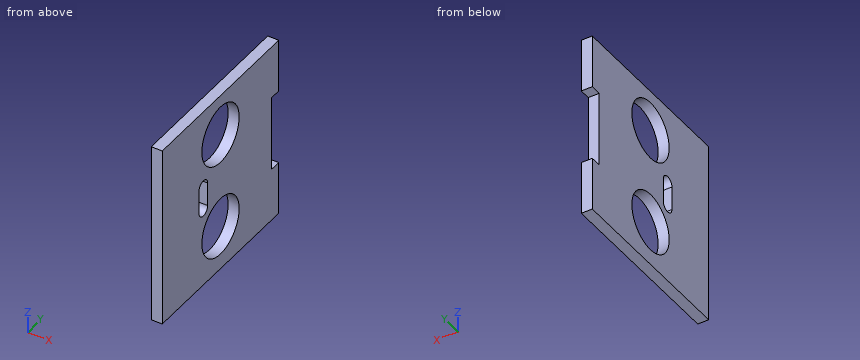
```python
from build123d import *

# Parameters (mm, degrees)
BOSS_EXTRUDE1_DEPTH = 3
SKETCH2_R           = 8
CUT_EXTRUDE1_DEPTH  = 36.482389998


with BuildPart() as part:
    # Sketch1 → Boss-Extrude1 (new body)
    with BuildSketch(Plane(origin=(0, 0, 0), x_dir=(0, 0, -1), z_dir=(1, 0, 0))):
        Polygon((-25, 25), (-10.35, 25), (-10.35, 22), (10.35, 22), (10.35, 25), (25, 25), (25, -25), (-25, -25), align=None)
    extrude(amount=BOSS_EXTRUDE1_DEPTH)

    # Sketch2 → Cut-Extrude1 (cut, through all)
    with BuildSketch(Plane(origin=(3, 0, 0), x_dir=(0, 0, -1), z_dir=(1, 0, 0))):
        with Locations((-13.73, 0)):
            Circle(SKETCH2_R)
        with Locations((12.77, 0)):
            Circle(SKETCH2_R)
        with BuildLine():
            Line((-3.25, -5.5), (3.25, -5.5))
            ThreePointArc((3.25, -5.5), (5.1, -7.35), (3.25, -9.2))
            Line((3.25, -9.2), (-3.25, -9.2))
            ThreePointArc((-3.25, -9.2), (-5.1, -7.35), (-3.25, -5.5))
        make_face()
    extrude(amount=-CUT_EXTRUDE1_DEPTH, mode=Mode.SUBTRACT)


solid = part.part
```
CAD build for the part. Positions are in the model's coordinates, mm. Round coordinates to 2 decimals unless told otherwise and drop trailing zeros. Loops run counter-clockwise (first coordinate to the right, second up) from the corner with the lowest first, then second, coordinate; pieces in that order, holes last. Notation, with made-up numbers: M 78,-5.75 L 126,-5.75 A30 ccw 126,28.25 Z; hole C 35.25,85 d11. An arc over 180 degrees is marked long. Return JSON: item names as keys, results as strings. Group by question number.
(1) Saw through at C-C, the plane x = 1.7. List the corners of the cut face in (y, z), and give its area (3 significant figures).
(2) Saw through at B-B, the plane y = 0. List the corners of the cut face in (x, z).
(3) Saw through at A-A, the plane z = 2.5. List the corners of the cut face in (x, y), and give its area (3 significant figures).
(4) Drop flat-ended pins along their axis: P1, Ø4, axis at y = 3, z = -6.5, coming from the -X side; P2, Ø1.5, axis at x = 1, z = 4.5, coming from the +Y side. Give the stop position or say it passes through.
(5) Saw through at D-D, the plane y = -7.35. List the corners of the cut face in (x, z).
(6) Wall check: probe 1 along Y at (x, z) = (1.8, 2); probe 2 along Z at (x, y) = (1.05, -1); probe 3 along Z at (x, y) = (1.3, 4). Give the ranges that are in metal, low to high. Write a range as [from, to].
Answer list:
{
 "1": {"outline": "M -25,-25 L 25,-25 L 25,-10.35 L 22,-10.35 L 22,10.35 L 25,10.35 L 25,25 L -25,25 Z; hole M -9.2,-3.25 A1.85 ccw -5.5,-3.25 L -5.5,3.25 A1.85 ccw -9.2,3.25 Z; hole C 0,-12.77 d16; hole C 0,13.73 d16", "area": "2,000 mm2"},
 "2": {"outline": "M 0,-25 L 3,-25 L 3,-20.77 L 0,-20.77 Z; M 0,-4.77 L 3,-4.77 L 3,5.73 L 0,5.73 Z; M 0,21.73 L 3,21.73 L 3,25 L 0,25 Z"},
 "3": {"outline": "M 0,-25 L 3,-25 L 3,-9.2 L 0,-9.2 Z; M 0,-5.5 L 3,-5.5 L 3,22 L 0,22 Z", "area": "130 mm2"},
 "4": {"P1": "x = 0", "P2": "y = 22"},
 "5": {"outline": "M 0,-25 L 3,-25 L 3,-15.93 L 0,-15.93 Z; M 0,-9.61 L 3,-9.61 L 3,-5.1 L 0,-5.1 Z; M 0,5.1 L 3,5.1 L 3,10.57 L 0,10.57 Z; M 0,16.89 L 3,16.89 L 3,25 L 0,25 Z"},
 "6": {"probe 1": "[-25, -9.2], [-5.5, 22]", "probe 2": "[-25, -20.71], [-4.83, 5.79], [21.67, 25]", "probe 3": "[-25, -19.7], [-5.84, 6.8], [20.66, 25]"}
}
